from build123d import *

# Parameters (mm, degrees)
SKETCH1_R                       = 60.96
BILLET_DEPTH                    = 5.842
SKETCH4_R                       = 0.7493
FIRST_KEROSENE_OUTLET_DEPTH     = 88.140881336
PRIMARY_HOLES_COUNT             = 6
SECOND_START                    = -5.842
SECOND_RING_OUTLINE_R           = 0.7493
SECOND_RING_DEPTH               = 5.842
THIRD_START                     = -5.842
THIRD_RING_OUTLINE_R            = 0.7493
THIRD_RING_DEPTH                = 5.842
SKETCH18_RX                     = 46.67504
SKETCH18_RY                     = 22.225
KEROSENE_WELL_DEPTH             = 2.032
SKETCH17_R                      = 6.35
BOSS_EXTRUDE1_DEPTH             = 2.54
BOSS_EXTRUDE1_DIRECTION_2_REACH = 88.408
SKETCH21_R                      = 6.35
CUT_EXTRUDE1_DEPTH              = 2.54
SKETCH32_R                      = 55.7149
SKETCH32_R_2                    = 51.6509
CUT_EXTRUDE5_DEPTH              = 2.6924
SKETCH20_R                      = 1.190625
CUT_EXTRUDE6_DEPTH              = 2.54


# Read off the part's stored shape, not the designer's step: Second ring, Third Ring
with BuildPart() as part:
    # Sketch1 → Billet (new body)
    with BuildSketch(Plane(origin=(0, 0, 0), x_dir=(1, 0, 0), z_dir=(0, 1, 0))):
        with Locations(Location((0, 0, 0), (0, 0, 270))):
            Circle(SKETCH1_R)
    extrude(amount=-BILLET_DEPTH)

    # Sketch4 → First Kerosene Outlet (cut, symmetric)
    with BuildSketch(Plane(origin=(0, -12.7, 0), x_dir=(1, 0, 0), z_dir=(0, 1, 0))):
        with Locations(Location((8.9916, 0, 0), (0, 0, 270))):
            Circle(SKETCH4_R)
        with Locations(Location((13.4874, 0, 0), (0, 0, 270))):
            Circle(SKETCH4_R)
        with Locations(Location((17.9832, 0, 0), (0, 0, 270))):
            Circle(SKETCH4_R)
    first_kerosene_outlet = extrude(amount=FIRST_KEROSENE_OUTLET_DEPTH, both=True, mode=Mode.SUBTRACT)

    # Primary Holes: First Kerosene Outlet ×6 about axis
    primary_holes_axis = Axis((0, 0, 0), (0, 1, 0))
    for i in range(1, PRIMARY_HOLES_COUNT):
        add(first_kerosene_outlet.rotate(primary_holes_axis, i * 360 / PRIMARY_HOLES_COUNT), mode=Mode.SUBTRACT)

    # Second ring outline → Second ring (cut)
    with BuildSketch(Plane(origin=(0, 0, 0), x_dir=(1, 0, 0), z_dir=(0, 1, 0)).offset(SECOND_START)):
        with Locations((11.680431031, 6.7437)):
            Circle(SECOND_RING_OUTLINE_R)
        with Locations((0, 13.4874)):
            Circle(SECOND_RING_OUTLINE_R)
        with Locations((-11.680431031, 6.7437)):
            Circle(SECOND_RING_OUTLINE_R)
        with Locations((-11.680431031, -6.7437)):
            Circle(SECOND_RING_OUTLINE_R)
        with Locations((0, -13.4874)):
            Circle(SECOND_RING_OUTLINE_R)
        with Locations((11.680431031, -6.7437)):
            Circle(SECOND_RING_OUTLINE_R)
    extrude(amount=SECOND_RING_DEPTH, mode=Mode.SUBTRACT)

    # Third Ring outline → Third Ring (cut)
    with BuildSketch(Plane(origin=(0, 0, 0), x_dir=(1, 0, 0), z_dir=(0, 1, 0)).offset(THIRD_START)):
        with Locations((17.370437319, 4.654394652)):
            Circle(THIRD_RING_OUTLINE_R)
        with Locations((15.573908041, 8.9916)):
            Circle(THIRD_RING_OUTLINE_R)
        with Locations((12.716042667, 12.716042667)):
            Circle(THIRD_RING_OUTLINE_R)
        with Locations((4.654394652, 17.370437319)):
            Circle(THIRD_RING_OUTLINE_R)
        with Locations((0, 17.9832)):
            Circle(THIRD_RING_OUTLINE_R)
        with Locations((-4.654394652, 17.370437319)):
            Circle(THIRD_RING_OUTLINE_R)
        with Locations((-12.716042667, 12.716042667)):
            Circle(THIRD_RING_OUTLINE_R)
        with Locations((-15.573908041, 8.9916)):
            Circle(THIRD_RING_OUTLINE_R)
        with Locations((-17.370437319, 4.654394652)):
            Circle(THIRD_RING_OUTLINE_R)
        with Locations((-17.370437319, -4.654394652)):
            Circle(THIRD_RING_OUTLINE_R)
        with Locations((-15.573908041, -8.9916)):
            Circle(THIRD_RING_OUTLINE_R)
        with Locations((-12.716042667, -12.716042667)):
            Circle(THIRD_RING_OUTLINE_R)
        with Locations((-4.654394652, -17.370437319)):
            Circle(THIRD_RING_OUTLINE_R)
        with Locations((0, -17.9832)):
            Circle(THIRD_RING_OUTLINE_R)
        with Locations((4.654394652, -17.370437319)):
            Circle(THIRD_RING_OUTLINE_R)
        with Locations((12.716042667, -12.716042667)):
            Circle(THIRD_RING_OUTLINE_R)
        with Locations((15.573908041, -8.9916)):
            Circle(THIRD_RING_OUTLINE_R)
        with Locations((17.370437319, -4.654394652)):
            Circle(THIRD_RING_OUTLINE_R)
    extrude(amount=THIRD_RING_DEPTH, mode=Mode.SUBTRACT)

    # Sketch18 → Kerosene Well (cut)
    with BuildSketch(Plane(origin=(0, 0, 0), x_dir=(1, 0, 0), z_dir=(0, 1, 0))):
        with Locations(Location((0, 0), (0, 0, -180))):
            Ellipse(SKETCH18_RX, SKETCH18_RY)
    extrude(amount=-KEROSENE_WELL_DEPTH, mode=Mode.SUBTRACT)

    # Sketch17 → Boss-Extrude1 (add)
    with BuildSketch(Plane(origin=(0, 0, 0), x_dir=(1, 0, 0), z_dir=(0, 1, 0))):
        with Locations(Location((0, 0, 0), (0, 0, 270))):
            Circle(SKETCH17_R)
    extrude(amount=BOSS_EXTRUDE1_DEPTH)

    # Sketch17 → Boss-Extrude1 direction 2 (add, up to next)
    with BuildSketch(Plane(origin=(0, 0, 0), x_dir=(1, 0, 0), z_dir=(0, 1, 0)), mode=Mode.PRIVATE) as boss_extrude1_direction_2_sk1:
        with Locations(Location((0, 0, 0), (0, 0, 270))):
            Circle(SKETCH17_R)
    boss_extrude1_direction_2_tool1 = extrude(boss_extrude1_direction_2_sk1.sketch, amount=-BOSS_EXTRUDE1_DIRECTION_2_REACH, mode=Mode.PRIVATE) - part.part
    add(boss_extrude1_direction_2_tool1.solids().sort_by_distance((0, 0, 0))[0])

    # Sketch21 → Cut-Extrude1 (cut)
    with BuildSketch(Plane(origin=(0, 2.54, 0), x_dir=(1, 0, 0), z_dir=(0, 1, 0))):
        with Locations(Location((0, 0, 0), (0, 0, 270))):
            Circle(SKETCH21_R)
    extrude(amount=-CUT_EXTRUDE1_DEPTH, mode=Mode.SUBTRACT)

    # Sketch32 → Cut-Extrude5 (cut)
    with BuildSketch(Plane.XZ.offset(5.842)):
        with Locations(Location((0, 0, 0), (0, 0, 270))):
            Circle(SKETCH32_R)
        with Locations(Location((0, 0, 0), (0, 0, 270))):
            Circle(SKETCH32_R_2, mode=Mode.SUBTRACT)
    extrude(amount=-CUT_EXTRUDE5_DEPTH, mode=Mode.SUBTRACT)

    # Sketch20 → Cut-Extrude6 (cut)
    with BuildSketch(Plane(origin=(0, 0, 0), x_dir=(1, 0, 0), z_dir=(0, 1, 0))):
        with Locations(Location((0, 25.4, 0), (0, 0, 270))):
            Circle(SKETCH20_R)
        with Locations(Location((0, -25.4, 0), (0, 0, 90))):
            Circle(SKETCH20_R)
        with Locations(Location((0, 44.45, 0), (0, 0, 270))):
            Circle(SKETCH20_R)
        with Locations(Location((0, -44.45, 0), (0, 0, 90))):
            Circle(SKETCH20_R)
    extrude(amount=-CUT_EXTRUDE6_DEPTH, mode=Mode.SUBTRACT)


solid = part.part
Model file for the job. Use its own axes, mm. A direction names the side the tool comes from. Round coordinates to 2 decimals unless told otherwise and drop trailing zeros. Loops run counter-clockwise (first coordinate to the right, second up) from the corner with the lowest first, then second, coordinate; pieces in that order, holes last.
1. Wall check: probe 1 along Z at (x, y) = (-18, -3.1); probe 2 along Z at (x, y) = (25, -4.8); probe 3 along Z at (x, y) = (-2, -4.3). Give the ranges that are in metal, low to high.
Check values:
probe 1: z = -58.24 to -5.06, -4.25 to -0.75, 0.75 to 4.25, 5.06 to 58.24
probe 2: z = -55.6 to -49.79, -45.2 to 45.2, 49.79 to 55.6
probe 3: z = -60.93 to -55.68, -51.61 to 51.61, 55.68 to 60.93
2. Band-saw the part on B-B, the plane z = -39. List the corners of the cut face in (x, y), and give its area (3 significant figures).
Check values:
outline: (-46.85, -5.84) - (-39.79, -5.84) - (-39.79, -3.15) - (-33.86, -3.15) - (-33.86, -5.84) - (33.86, -5.84) - (33.86, -3.15) - (39.79, -3.15) - (39.79, -5.84) - (46.85, -5.84) - (46.85, 0) - (-46.85, 0) - close
area: 516 mm2
3. Band-saw the part on A-A, the plane y = -1.15. Count the separate pieces of the cut face and the enclosed holes in it, and give its area (3 significant figures).
Check values:
separate pieces: 2
enclosed holes: 5
area: 8,520 mm2
4. Tool access for faces 1 (the flat face through (-10, -2.032, 0)), 2 (the flat face through (-49, -5.842, 27)), 3 (the cylindrical face through (-21.339, -4.515, -51.466)): list every direction of +Z, -Z, +X, -X, +Y, -Y with a clear straight run to the whole face (end or side of a thin tool).
Check values:
face 1: +Y
face 2: +Z, -Z, +X, -X, -Y
face 3: -Y
5. Drop flat-ended pins along their axis: P1, Ø1.5, axis at y = -0.5, z = 20, coming from the +X side; P2, Ø3, axis at x = -40.5, y = -3, coming from the +Z side; P3, Ø1.9, axis at x = -12.72, z = -12.72, coming from the +Y side. Give the stop position or say it passes through.
Check values:
P1: stops at x = 57.84
P2: stops at z = 46.85
P3: stops at y = -2.03
6. Mould opens along X. For faces 4 (the cylindrical face through (51.21, -4.51, 6.72)), 5 (the flat face through (-13, 0, 26)), 6 (the cylindrical face through (60.44, -2.88, -7.94)) say: +X half, -X half, draft (parallel to the pull), parting line (faces both ways), or undercut.
Check values:
face 4: undercut
face 5: draft
face 6: parting line
